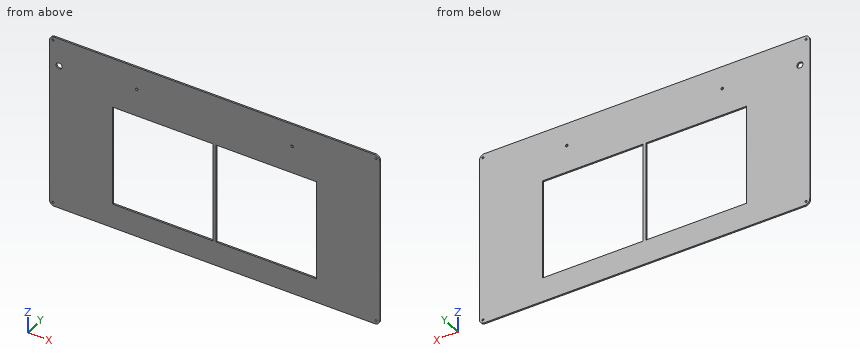
from build123d import *

# Parameters (mm, degrees)
SKETCH_1_R      = 2
SKETCH_1_R_2    = 6
SKETCH_1_R_3    = 2.5
EXTRUDE_1_DEPTH = 3


with BuildPart() as part:
    # 草图1 → 凸台-拉伸1 (new body)
    with BuildSketch(Plane(origin=(0, 0, 0), x_dir=(1, 0, 0), z_dir=(0, 1, 0))):
        with BuildLine():
            Line((630, 344), (20, 344))
            Line((20, 344), (16, 344))
            ThreePointArc((16, 344), (8.928932188, 341.071067812), (6, 334))
            Line((6, 334), (6, 330))
            Line((6, 330), (6, 20))
            Line((6, 20), (6, 16))
            ThreePointArc((6, 16), (8.928932188, 8.928932188), (16, 6))
            Line((16, 6), (20, 6))
            Line((20, 6), (630, 6))
            Line((630, 6), (634, 6))
            ThreePointArc((634, 6), (641.071067812, 8.928932188), (644, 16))
            Line((644, 16), (644, 20))
            Line((644, 20), (644, 330))
            Line((644, 330), (644, 334))
            ThreePointArc((644, 334), (641.071067812, 341.071067812), (634, 344))
            Line((634, 344), (630, 344))
        make_face()
        with Locations(Location((13, 13, 0), (0, 0, 270))):
            Circle(SKETCH_1_R, mode=Mode.SUBTRACT)
        with Locations(Location((25, 60, 0), (0, 0, 270))):
            Circle(SKETCH_1_R_2, mode=Mode.SUBTRACT)
        with Locations(Location((175, 50, 0), (0, 0, 270))):
            Circle(SKETCH_1_R_3, mode=Mode.SUBTRACT)
        with Locations(Location((475, 50, 0), (0, 0, 270))):
            Circle(SKETCH_1_R_3, mode=Mode.SUBTRACT)
        with Locations(Location((637, 13, 0), (0, 0, 270))):
            Circle(SKETCH_1_R, mode=Mode.SUBTRACT)
        Polygon((322, 297), (322, 175), (322, 103), (128, 103), (128, 297), align=None, mode=Mode.SUBTRACT)
        with Locations(Location((13, 337, 0), (0, 0, 270))):
            Circle(SKETCH_1_R, mode=Mode.SUBTRACT)
        Polygon((522, 297), (522, 103), (328, 103), (328, 175), (328, 297), align=None, mode=Mode.SUBTRACT)
        with Locations(Location((637, 337, 0), (0, 0, 270))):
            Circle(SKETCH_1_R, mode=Mode.SUBTRACT)
    extrude(amount=-EXTRUDE_1_DEPTH)


solid = part.part
Source: CAD feature listing. Evaluate the final solid. Frame: model axes, mm. Give positions to 0.01 mm unless a question says otherwise; leave off trailing zeros. Order: outer loops, then holes, each group sorted by start corner. A loop starts at its lowest first (then second) coordinate and runs counter-clockwise, first axis right, second up. Notation, with made-up numbers: (23.25, 3.5) -> (60.25, 3.5) arc R26 ccw to (60.25, 35.5) -> close; hole circle Ø5 at (52, 15.5). An arc over 180 degrees is marked (long way). Write item = value, one per line.
Q1. Cut plane C-C, the plane y = -2.45. State how many separate pieces and enclosed holes the cut face has, and give its area (3 significant figures).
Data:
separate_pieces = 1
enclosed_holes = 9
area = 140,000 mm^2
Q2. Material intervals for line 1 (X direction, y = -0.45, z = -277); line 2 (Z direction, x = 289.5, y = -1.3); line 3 (Z direction, x = 637, y = -1.4), sorted ascending. Write a range as from..to.
Data:
line_1 = 6..128, 322..328, 522..644
line_2 = -344..-297, -103..-6
line_3 = -343.54..-339, -335..-15, -11..-6.46
Q3. Pin query (flat end, axial travel): pin 1 (2.5 mm diameter, centred on x = 13, z = -337, fed in from -Y). Return the tip coordinate at first contact, or that it passes through.
Data:
pin_1 = through
Q4. Cut plane A-A, the plane x = 189. Output: boundary loops of the cut face in (y, z), and give its area (3 significant figures).
Data:
outline = (-3, -344) -> (0, -344) -> (0, -297) -> (-3, -297) -> close; (-3, -103) -> (0, -103) -> (0, -6) -> (-3, -6) -> close
area = 432 mm^2
Q5. Cut plane B-B, the plane z = -60. Output: boundary loops of the cut face in (x, y).
Data:
outline = (6, -3) -> (19, -3) -> (19, 0) -> (6, 0) -> close; (31, -3) -> (644, -3) -> (644, 0) -> (31, 0) -> close
